Answer from the drawing. Dimensions are ordinates in mm from the lowest x, y and z of the part. A direction names the side the tool comes from. Give positions to 0.01 mm unless a question says otherwise; leave off trailing zeros. Write each loop counter-clockwise with the first axis right and the second up, starting at its lowest first coordinate (ties: lowest second). Pieces come first, ordered by that corner, then holes.
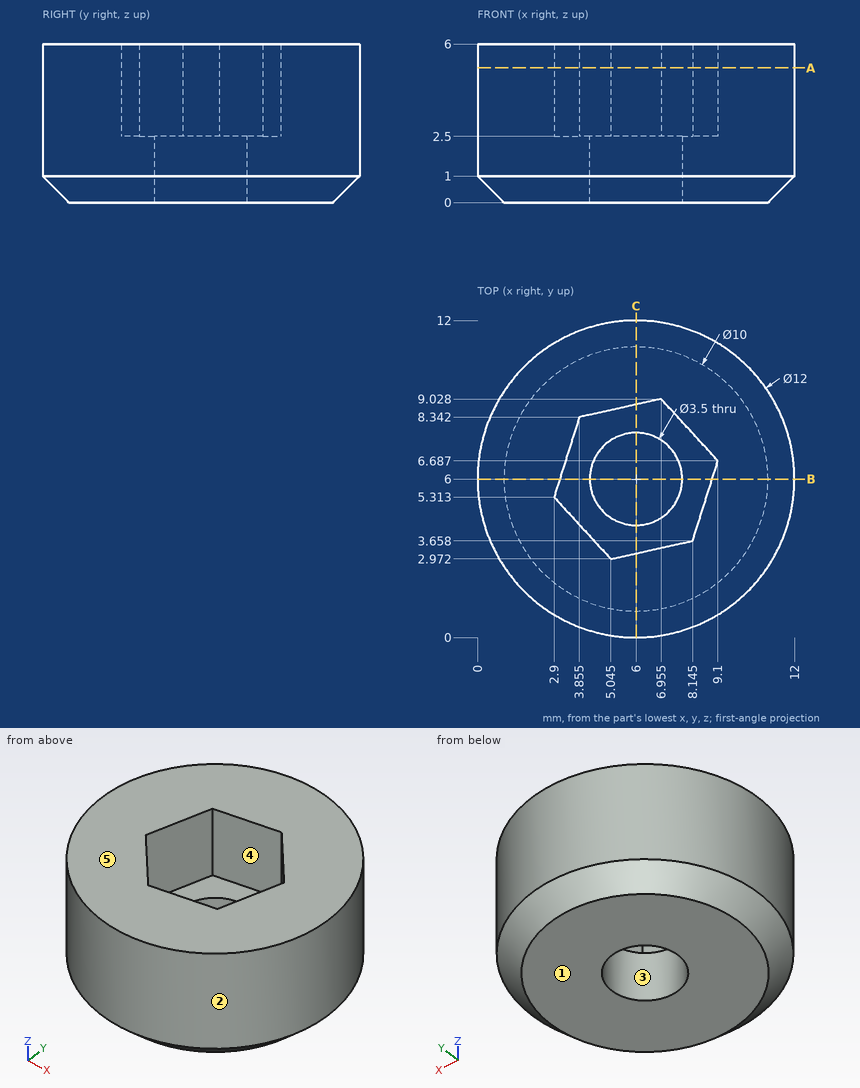
Item 1: Each of these flat-tipped pins is pushed along its axis until it touches: P1, Ø5.5, axis at x = 6, y = 6, coming from the -Z side; P2, Ø1, axis at y = 8.5, z = 4, coming from the -X side; P3, Ø2, axis at y = 3.5, z = 4, coming from the +X side. Where does it stop, or does it pass through?
Conclusion:
P1: stops at z = 0
P2: stops at x = 0.34
P3: stops at x = 11.81
Item 2: Consider probe 1 along Y at (x, z) = (6, 1.7); probe 2 along Z at (x, y) = (3.5, 5); probe 3 along X at (y, z) = (4.75, 4) (1 decimal). Determine where each line is inside the solid, lowest interval first.
Conclusion:
probe 1: y = 0 to 4.25, 7.75 to 12
probe 2: z = 0 to 2.5
probe 3: x = 0.1 to 3.4, 8.5 to 11.9
Item 3: A cutting plane is placed at C-C, the plane x = 6. Give the vertices of the cut face in (y, z).
Conclusion:
outline: (0, 1) - (1, 0) - (4.25, 0) - (4.25, 2.5) - (3.18, 2.5) - (3.18, 6) - (0, 6) - close; (7.75, 0) - (11, 0) - (12, 1) - (12, 6) - (8.82, 6) - (8.82, 2.5) - (7.75, 2.5) - close
Item 4: A cutting plane is placed at A-A, the plane z = 5.1. Give the vertices of the cut face in (x, y) (1 decimal).
Conclusion:
outline: circle Ø12 at (6, 6); hole (2.9, 5.3) - (5, 3) - (8.1, 3.7) - (9.1, 6.7) - (7, 9) - (3.9, 8.3) - close
Item 5: Determine the mould class of the marked faces 1, 2 and 3 for opening direction Y: pulls with the +Y half, pulls with the -Y half, needs draft (parallel to the pull), parting line crosses it, or undercut.
Conclusion:
face 1: needs draft
face 2: parting line crosses it
face 3: undercut
Item 6: A cutting plane is placed at B-B, the plane y = 6. Give the vertices of the cut face in (x, z).
Conclusion:
outline: (0, 1) - (1, 0) - (4.25, 0) - (4.25, 2.5) - (3.12, 2.5) - (3.12, 6) - (0, 6) - close; (7.75, 0) - (11, 0) - (12, 1) - (12, 6) - (8.88, 6) - (8.88, 2.5) - (7.75, 2.5) - close
Item 7: Which of the six approach directions +Z, -Z, +X, -X, +Y, -Y give full straight-line access (tool end or side, diameter ignored) to the marked faces 4 and 5?
Conclusion:
face 4: +Z
face 5: +Z, +X, -X, +Y, -Y
